Part model, mm, in its own coordinate system. Face numbers are marked on the shaded views. A direction names the side the tool comes from. Round coordinates to 2 decimals unless told otherwise and drop trailing zeros. Loops run counter-clockwise (first coordinate to the right, second up) from the corner with the lowest first, then second, coordinate; pieces in that order, holes last.
(1) Cut at A-A on z = 8. List the corners of the cut face in (x, y), then the cut area to 3 significant figures.
(2) Probe probe 1 along Z at (x, y) = (3, -0.5); probe 2 along Y at (x, z) = (1.75, 25.5); probe 3 along X at (y, z) = (-1.5, 8). List the from-to ranges inside material, lowest first.
(3) Flat gauge pins, fed straight in: pin 1 (1 mm diameter, centred on y = -2, z = 8.5, fed in from -X); pin 2 (4 mm diameter, centred on y = 0, z = 5, fed in from -X). Where does each tip first touch, or does it go through?
(4) Tool access for the marked faces 4 and 5: list every direction of +Z, -Z, +X, -X, +Y, -Y with a clear straight run to the whole face (end or side of a thin tool).
(5) Cut at B-B on x = 1.5. List the corners of the cut face in (y, z), then the cut area to 3 significant figures.
(6) Cut at C-C on y = -3.75. List the corners of the cut face in (x, z).
(7) Cut at D-D on x = 4.5. List the corners of the cut face in (y, z), then the cut area to 3 significant figures.
(8) Mould opens along X. For the marked faces 1, 2 and 3 say: +X half, -X half, draft (parallel to the pull), parting line (faces both ways), or undercut.
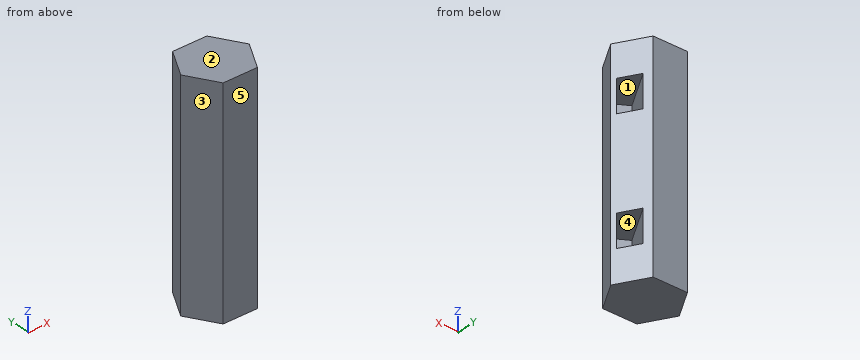
from build123d import *

# Parameters (mm, degrees)
BOSS_EXTRU_1_DEPTH      = 34
ENL_V_MAT_EXTRU_1_DEPTH = 5


with BuildPart() as part:
    # Esquisse1 → Boss.-Extru.1 (new body)
    with BuildSketch(Plane.XY):
        Polygon((-2.690598923, 4.660254038), (-5.381197846, 0), (-2.690598923, -4.660254038), (2.690598923, -4.660254038), (5.381197846, 0), (2.690598923, 4.660254038), align=None)
    extrude(amount=BOSS_EXTRU_1_DEPTH)

    # Esquisse2 → Enlèv. mat.-Extru.1 (cut)
    with BuildSketch(Plane.XY.offset(5)):
        Polygon((3.657319172, 4.134662626), (-0.392671517, -2.880127019), (2.118802154, -4.330127019), (6.168792843, 2.684662626), align=None)
    enl_v_mat_extru_1 = extrude(amount=ENL_V_MAT_EXTRU_1_DEPTH, mode=Mode.SUBTRACT)

    # Symétrie1: Enlèv. mat.-Extru.1 across plane
    add(enl_v_mat_extru_1.mirror(Plane(origin=(0, 0, 17), x_dir=(1, 0, 0), z_dir=(0, 0, -1))), mode=Mode.SUBTRACT)


solid = part.part
Final values:
1. outline: (-5.38, 0) - (-2.69, -4.66) - (2.69, -4.66) - (5.38, 0) - (5, 0.66) - (2.12, -4.33) - (-0.39, -2.88) - (3.33, 3.56) - (2.69, 4.66) - (-2.69, 4.66) - close
1. area: 56.1 mm2
2. probe 1: z = 0 to 5, 10 to 24, 29 to 34
2. probe 2: y = -4.66 to -4.12, 0.83 to 4.66
2. probe 3: x = -4.52 to 0.4, 3.75 to 4.52
3. pin 1: stops at x = -4.52
3. pin 2: stops at x = -5.38
4. face 4: none
4. face 5: +Z, -Z, +X, -X, -Y
5. outline: (-4.66, 0) - (4.66, 0) - (4.66, 34) - (-4.66, 34) - close; hole (-3.97, 5) - (0.4, 5) - (0.4, 10) - (-3.97, 10) - close; hole (-3.97, 24) - (0.4, 24) - (0.4, 29) - (-3.97, 29) - close
5. area: 273 mm2
6. outline: (-3.22, 0) - (3.22, 0) - (3.22, 34) - (-3.22, 34) - close; hole (1.11, 5) - (2.45, 5) - (2.45, 10) - (1.11, 10) - close; hole (1.11, 24) - (2.45, 24) - (2.45, 29) - (1.11, 29) - close
7. outline: (-1.53, 0) - (1.53, 0) - (1.53, 5) - (-0.21, 5) - (-0.21, 10) - (1.53, 10) - (1.53, 24) - (-0.21, 24) - (-0.21, 29) - (1.53, 29) - (1.53, 34) - (-1.53, 34) - close
7. area: 86.5 mm2
8. face 1: undercut
8. face 2: draft
8. face 3: -X half
